from build123d import *

# Parameters (mm, degrees)
F1_DEPTH = 3.81
F2_R     = 2.786775
F2_R_2   = 2.454424
F3_DEPTH = 6.35
F4_W     = 3.428999
F4_H     = 2.867069
F5_DEPTH = 5.08
F6_R     = 2.706702
F7_DEPTH = 2.54


with BuildPart() as f1:
    # F0 (on Top) → F1 (new body)
    with BuildSketch(Plane.XY):
        Polygon((14.661641, 0.299343), (7.071582, 12.847025), (-7.590059, 12.547683), (-14.661641, -0.299343), (-7.071582, -12.847025), (7.590059, -12.547683), align=None)
    extrude(amount=F1_DEPTH)

    # F2 (on face) → F3 (join)
    with BuildSketch(Plane.XY.offset(3.81)):
        with Locations((-5.619749, 6.562192)):
            Circle(F2_R)
        with Locations((5.048249, 8.448053)):
            Circle(F2_R_2)
        Polygon((8.512636, -3.522729), (8.367075, 3.606768), (2.265531, -0.08404), align=None)
    extrude(amount=F3_DEPTH)

    # F4 (on face) → F5 (cut)
    with BuildSketch(Plane.XY.offset(3.81)):
        with Locations((-6.953249, -1.433534)):
            Rectangle(F4_W, F4_H)
    extrude(amount=-F5_DEPTH, mode=Mode.SUBTRACT)

    # F6 (on face) → F7 (cut)
    with BuildSketch(Plane.XY.offset(3.81)):
        with Locations((-4.522542, -6.642293)):
            Circle(F6_R)
    extrude(amount=-F7_DEPTH, mode=Mode.SUBTRACT)


solid = f1.part
Source: CAD feature listing. Evaluate the final solid. Frame: model axes, mm. A direction names the side the tool comes from. Coordinates: 2 decimals unless noted, no trailing zeros. Loops run counter-clockwise (first coordinate to the right, second up) from the corner with the lowest first, then second, coordinate; pieces in that order, holes last. Notation, with made-up numbers: (54.25, 13.25) - (93.25, 13.25) arc R12 cw to (93.25, 25.25) - close; hole circle Ø11 at (1.5, 27.5). An arc over 180 degrees is marked (long way). One line per question, with ' | ' between items.
1) Section B-B, the plane y = -1.5. Return loops of the section in (x, z), then the cut area to 3 significant figures.
Report:
outline: (-13.94, 0) - (-8.67, 0) - (-8.67, 3.81) - (-13.94, 3.81) - close; (-5.24, 0) - (13.67, 0) - (13.67, 3.81) - (8.47, 3.81) - (8.47, 10.16) - (4.84, 10.16) - (4.84, 3.81) - (-5.24, 3.81) - close | area: 115 mm²
2) First-contact query: P1, Ø3, axis at y = -2, z = 2, coming from the -X side; P2, Ø6, axis at x = -5, y = -7, coming from the +Z side; P3, Ø2, axis at x = 1, z = 9, coming from the -Y side; P4, Ø0.9, axis at y = -2, z = 2, coming from the +X side. Flat tips, straight axial feed; report the tip coordinate or a pass-through.
Report:
P1: stops at x = -14.54 | P2: stops at z = 3.81 | P3: passes through | P4: stops at x = 13.64
3) Section A-A, the plane z = 2.25. Return loops of the section in (x, y), then the cut area to 3 significant figures.
Report:
outline: (-14.66, -0.3) - (-7.07, -12.85) - (7.59, -12.55) - (14.66, 0.3) - (7.07, 12.85) - (-7.59, 12.55) - close; hole (-8.67, -2.87) - (-5.24, -2.87) - (-5.24, 0) - (-8.67, 0) - close; hole circle Ø5.41 at (-4.52, -6.64) | area: 526 mm²
4) Set-up query: faces 4 (the face through (5.36, 1.79, 6.94)), 5 (the face through (-7.227, -6.523, 2.558)), 6 (the face through (5.35, -1.78, 6.94)). Return all of +Z, -Z, +X, -X, +Y, -Y with unobstructed straight access to the full face (end or side cutting, diameter ignored); none if empty.
Report:
face 4: +Z, -X | face 5: +Z | face 6: +Z, -X, -Y
5) Line query: line 1 along Z through (x, y) = (10.25, 1.25); line 2 along X through (y, z) = (-2.25, 3.5); line 3 along Z through (x, y) = (-4, -6). Output: solid intervals per line, ascending.
Report:
line 1: z = 0 to 3.81 | line 2: x = -13.48 to -8.67, -5.24 to 13.26 | line 3: z = 0 to 1.27
6) Section C-C, the plane z = 6.5. Return loops of the section in (x, y), then the cut area to 3 significant figures.
Report:
outline: circle Ø5.57 at (-5.62, 6.56); (2.27, -0.08) - (8.51, -3.52) - (8.37, 3.61) - close; circle Ø4.91 at (5.05, 8.45) | area: 65.3 mm²
7) Pull-direction query (X, two-part tool) for faces 1 (the face through (-6, 7, 10.16)), 2 (the face through (11.08, -6.21, 1.88)), 3 (the face through (-7, 0, 2)); classes: released by +X, released by -X, zero draft, split by the parting line, or undercut.
Report:
face 1: zero draft | face 2: released by +X | face 3: undercut
8) Section D-D, the plane x = 8. Return loops of the section in (y, z), then the cut area to 3 significant figures.
Report:
outline: (-11.8, 0) - (11.31, 0) - (11.31, 3.81) - (3.38, 3.81) - (3.38, 10.16) - (-3.24, 10.16) - (-3.24, 3.81) - (-11.8, 3.81) - close | area: 130 mm²
